from build123d import *

# Parameters (mm, degrees)
ESQUISSE1_W             = 305
ESQUISSE1_H             = 280
BOSS_EXTRU_1_DEPTH      = 5
ESQUISSE2_W             = 90
ESQUISSE2_H             = 123.7
ENL_V_MAT_EXTRU_1_DEPTH = 5
ESQUISSE3_R             = 1.5
ENL_V_MAT_EXTRU_2_DEPTH = 415.065212255
ESQUISSE4_R             = 1.6
ESQUISSE4_W             = 7.3
ESQUISSE4_H             = 28
ENL_V_MAT_EXTRU_3_DEPTH = 415.065212255
ESQUISSE5_R             = 8
ESQUISSE5_R_2           = 1
ENL_V_MAT_EXTRU_4_DEPTH = 415.065212255


with BuildPart() as part:
    # Esquisse1 → Boss.-Extru.1 (new body)
    with BuildSketch(Plane.XY):
        with Locations((152.5, 140)):
            Rectangle(ESQUISSE1_W, ESQUISSE1_H)
    extrude(amount=BOSS_EXTRU_1_DEPTH)

    # Esquisse2 → Enlèv. mat.-Extru.1 (cut)
    with BuildSketch(Plane.XY.offset(5)):
        with Locations((198.5, 144.37)):
            Rectangle(ESQUISSE2_W, ESQUISSE2_H)
    extrude(amount=-ENL_V_MAT_EXTRU_1_DEPTH, mode=Mode.SUBTRACT)

    # Esquisse3 → Enlèv. mat.-Extru.2 (cut, through all)
    with BuildSketch(Plane(origin=(0, 0, 0), x_dir=(-1, 0, 0), z_dir=(0, 0, -1))):
        with Locations((-15, 92.5)):
            Circle(ESQUISSE3_R)
        with Locations((-35, 92.5)):
            Circle(ESQUISSE3_R)
        with Locations((-35, 186.5)):
            Circle(ESQUISSE3_R)
        with Locations((-15, 186.5)):
            Circle(ESQUISSE3_R)
        with Locations((-255, 249.4)):
            Circle(ESQUISSE3_R)
        with Locations((-255, 269.4)):
            Circle(ESQUISSE3_R)
        with Locations((-255.5, 10)):
            Circle(ESQUISSE3_R)
        with Locations((-255.5, 30)):
            Circle(ESQUISSE3_R)
    extrude(amount=-ENL_V_MAT_EXTRU_2_DEPTH, mode=Mode.SUBTRACT)

    # Esquisse4 → Enlèv. mat.-Extru.3 (cut, through all)
    with BuildSketch(Plane.XY.offset(5)):
        with Locations((139.85, 159.5)):
            Circle(ESQUISSE4_R)
        with Locations((139.85, 122.5)):
            Circle(ESQUISSE4_R)
        with Locations((279.35, 82.5)):
            Circle(ESQUISSE4_R)
        with Locations((279.35, 45.5)):
            Circle(ESQUISSE4_R)
        with Locations((279.35, 121.5)):
            Circle(ESQUISSE4_R)
        with Locations((279.35, 158.5)):
            Circle(ESQUISSE4_R)
        with Locations((279.35, 197.5)):
            Circle(ESQUISSE4_R)
        with Locations((279.35, 234.5)):
            Circle(ESQUISSE4_R)
        with Locations((279.35, 64)):
            Rectangle(ESQUISSE4_W, ESQUISSE4_H)
        with Locations((279.35, 140)):
            Rectangle(ESQUISSE4_W, ESQUISSE4_H)
        with Locations((279.35, 216)):
            Rectangle(ESQUISSE4_W, ESQUISSE4_H)
        with Locations((139.85, 141)):
            Rectangle(ESQUISSE4_W, ESQUISSE4_H)
    extrude(amount=-ENL_V_MAT_EXTRU_3_DEPTH, mode=Mode.SUBTRACT)

    # Esquisse5 → Enlèv. mat.-Extru.4 (cut, through all)
    with BuildSketch(Plane.XY.offset(5)):
        with Locations((95, 127)):
            Circle(ESQUISSE5_R)
        with Locations((95, 154)):
            Circle(ESQUISSE5_R)
        with Locations((87.715791554, 120.451688458)):
            Circle(ESQUISSE5_R_2)
        with Locations((87.284208446, 160.451688458)):
            Circle(ESQUISSE5_R_2)
        with Locations((102.284208446, 160.548311542)):
            Circle(ESQUISSE5_R_2)
        with Locations((102.715791554, 120.548311542)):
            Circle(ESQUISSE5_R_2)
    extrude(amount=-ENL_V_MAT_EXTRU_4_DEPTH, mode=Mode.SUBTRACT)


solid = part.part
Can you work these out from the model? Positions are in its coordinate system, mm. Round coordinates to 2 decimals unless told otherwise and drop trailing zeros. Order: outer loops, then holes, each group sorted by start corner. A loop starts at its lowest first (then second) coordinate and runs counter-clockwise, first axis right, second up. Notation, with made-up numbers: (18, 14.25) -> (76, 14.25) arc R26 cw to (76, 37.25) -> close; hole circle Ø5 at (37, 12.5). An arc over 180 degrees is marked (long way). Write each question's results on one line, items separated by ' | '. Start each with the question number.
Item 1: Thinking about a two-plate mould opening in Y: for faces 1 (the cylindrical face through (93.27, 146.19, 2.54)), 2 (the flat face through (150, 142, 0)), which applies, +Y half, -Y half, draft (parallel to the pull), parting line (faces both ways), or undercut?
Item 2: If we section it at D-D, the plane x = 186.5: Write out the boundary of the cut face in (y, z).
Item 3: Please list where these lines run through material, in increasing order: L1, parallel to X at y = 92.5, z = 4; L2, parallel to Y at x = 35, z = 2.4; L3, parallel to Y at x = 95, z = 0.5.
Item 4: If we section it at B-B, the plane x = 95: Write out the boundary of the cut face in (y, z).
Item 5: If we section it at A-A, the plane y = 139: Write out the boundary of the cut face in (x, z), then the cut area to 3 significant figures.
Item 6: If we section it at C-C, the plane y = 58: Write out the boundary of the cut face in (x, z), then the cut area to 3 significant figures.
Results:
1) face 1: undercut | face 2: draft
2) outline: (0, 0) -> (82.52, 0) -> (82.52, 5) -> (0, 5) -> close; (206.22, 0) -> (280, 0) -> (280, 5) -> (206.22, 5) -> close
3) L1: x = 0 to 13.5, 16.5 to 33.5, 36.5 to 153.5, 243.5 to 305 | L2: y = 0 to 91, 94 to 185, 188 to 280 | L3: y = 0 to 119, 135 to 146, 162 to 280
4) outline: (0, 0) -> (119, 0) -> (119, 5) -> (0, 5) -> close; (135, 0) -> (146, 0) -> (146, 5) -> (135, 5) -> close; (162, 0) -> (280, 0) -> (280, 5) -> (162, 5) -> close
5) outline: (0, 0) -> (136.2, 0) -> (136.2, 5) -> (0, 5) -> close; (143.5, 0) -> (153.5, 0) -> (153.5, 5) -> (143.5, 5) -> close; (243.5, 0) -> (275.7, 0) -> (275.7, 5) -> (243.5, 5) -> close; (283, 0) -> (305, 0) -> (305, 5) -> (283, 5) -> close | area: 1,000 mm2
6) outline: (0, 0) -> (275.7, 0) -> (275.7, 5) -> (0, 5) -> close; (283, 0) -> (305, 0) -> (305, 5) -> (283, 5) -> close | area: 1,490 mm2
